Can you work these out from the model? Positions are in its coordinate system, mm. Face numbers are marked on the shaded views. A direction names the side the tool comes from. Coordinates: 2 decimals unless noted, no trailing zeros. Loops run counter-clockwise (first coordinate to the right, second up) from the corner with the lowest first, then second, coordinate; pieces in that order, holes last.
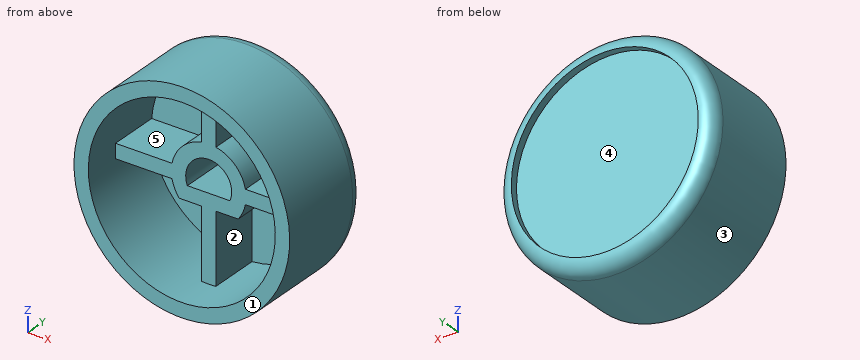
```python
from build123d import *

# Parameters (mm, degrees)
SKETCH1_R           = 15
BOSS_EXTRUDE1_DEPTH = 14.2
SHELL1_T            = -2
EXTRUDE_THIN2_DEPTH = 7
RIB1_REACH          = 25.043
SKETCH3_WALLS_W     = 2
SKETCH3_WALLS_H     = 57.886874488
CIRPATTERN1_COUNT   = 4
FILLET1_R           = 2
SKETCH4_R           = 13
CUT_EXTRUDE1_DEPTH  = 1


with BuildPart() as part:
    # Sketch1 → Boss-Extrude1 (new body)
    with BuildSketch(Plane(origin=(0, 0, 0), x_dir=(1, 0, 0), z_dir=(0, 1, 0))):
        with Locations(Location((0, 0, 0), (0, 0, 270))):
            Circle(SKETCH1_R)
    extrude(amount=-BOSS_EXTRUDE1_DEPTH)

    # Shell1
    shell1_openings = [part.faces().sort_by_distance(p)[0] for p in [
        (0, -14.2, 0),
    ]]
    offset(amount=SHELL1_T, openings=shell1_openings, kind=Kind.INTERSECTION)

    # Sketch2 → Extrude-Thin2 (add)
    with BuildSketch(Plane.XZ.offset(2)):
        with BuildLine():
            Line((-4.098780306, -3.2), (4.098780306, -3.2))
            ThreePointArc((4.098780306, -3.2), (0, 5.2), (-4.098780306, -3.2))
        make_face()
        with BuildLine():
            Line((-2.966479395, -1.2), (2.966479395, -1.2))
            ThreePointArc((2.966479395, -1.2), (0, 3.2), (-2.966479395, -1.2))
        make_face(mode=Mode.SUBTRACT)
    extrude(amount=EXTRUDE_THIN2_DEPTH)

    # Sketch3 walls → Rib1 (add, up to next)
    with BuildSketch(Plane.XZ.offset(9), mode=Mode.PRIVATE) as rib1_sk1:
        with Locations((0, -8.1)):
            Rectangle(SKETCH3_WALLS_W, SKETCH3_WALLS_H)
    rib1_tool1 = extrude(rib1_sk1.sketch, amount=-RIB1_REACH, mode=Mode.PRIVATE) - part.part
    rib1 = rib1_tool1.solids().sort_by_distance((0, -9, -8.1))[0]
    add(rib1)

    # CirPattern1: Rib1 ×4 about axis
    cirpattern1_axis = Axis((0, 0, 0), (0, 1, 0))
    for i in range(1, CIRPATTERN1_COUNT):
        add(rib1.rotate(cirpattern1_axis, i * 360 / CIRPATTERN1_COUNT))

    # Fillet1
    fillet1_edges = [part.edges().sort_by_distance(p)[0] for p in [
        (0, 0, -15),
    ]]
    fillet(fillet1_edges, radius=FILLET1_R)

    # Sketch4 → Cut-Extrude1 (cut)
    with BuildSketch(Plane(origin=(0, 0, 0), x_dir=(1, 0, 0), z_dir=(0, 1, 0))):
        with Locations(Location((0, 0, 0), (0, 0, 270))):
            Circle(SKETCH4_R)
    extrude(amount=-CUT_EXTRUDE1_DEPTH, mode=Mode.SUBTRACT)


solid = part.part
```
(1) I want a section at B-B on z = 0. Write out the boundary of the cut face in (x, y).
Check values:
outline: (-15, -14.2) - (-13, -14.2) - (-13, -9) - (-3.2, -9) - (-3.2, -2) - (3.2, -2) - (3.2, -9) - (13, -9) - (13, -14.2) - (15, -14.2) - (15, -2) arc R2 ccw to (13, 0) - (13, -1) - (-13, -1) - (-13, 0) arc R2 ccw to (-15, -2) - close
(2) I'm going to push flat-ended pins straight in: pin 1 (1.5 mm diameter, centred on x = 7.5, y = -12, fed in from +Z); pin 2 (13 mm diameter, centred on x = 6, z = -4.5, fed in from -Y); pin 3 (2 mm diameter, centred on x = -8.5, y = -4.5, fed in from -Z); pin 4 (8 mm diameter, centred on y = -2.5, z = 11.5, fed in from +X). Where does each tip first touch, or does it pass through?
Check values:
pin 1: stops at z = 13.4
pin 2: stops at y = -14.2
pin 3: stops at z = -12.99
pin 4: stops at x = 12.99
(3) Which directions (+Z, -Z, +X, -X, +Y, -Y) give clear straight access to the entire face, cutting with the end or side of a thin tool? Please do the marked faces 4 and 5.
Check values:
face 4: +Y
face 5: -Y
(4) I want a section at C-C on x = 0. Write out the boundary of the cut face in (y, z), then the cut area to 3 significant figures.
Check values:
outline: (-14.2, -15) - (-2, -15) arc R2 ccw to (0, -13) - (-1, -13) - (-1, 13) - (0, 13) arc R2 ccw to (-2, 15) - (-14.2, 15) - (-14.2, 13) - (-9, 13) - (-9, 3.2) - (-2, 3.2) - (-2, -1.2) - (-9, -1.2) - (-9, -13) - (-14.2, -13) - close
area: 232 mm2
(5) If we mould it in two halves opening along X, with no side actions, what happens to the marked faces 1, 2 and 3? For each: released by +X, released by -X, zero draft, split by the parting line, or undercut.
Check values:
face 1: zero draft
face 2: undercut
face 3: split by the parting line
(6) I want a section at A-A on y = -5. Write out the boundary of the cut face in (x, z), then the cut area to 3 significant figures.
Check values:
outline: circle Ø30 at (0, 0); hole (-12.96, -1) arc R13 ccw to (-1, -12.96) - (-1, -3.2) - (-4.1, -3.2) arc R5.2 cw to (-5.1, -1) - close; hole (-12.96, 1) - (-5.1, 1) arc R5.2 cw to (-1, 5.1) - (-1, 12.96) arc R13 ccw to start; hole (-2.97, -1.2) - (2.97, -1.2) arc R3.2 ccw (long way) to start; hole (1, -12.96) arc R13 ccw to (12.96, -1) - (5.1, -1) arc R5.2 cw to (4.1, -3.2) - (1, -3.2) - close; hole (1, 5.1) arc R5.2 cw to (5.1, 1) - (12.96, 1) arc R13 ccw to (1, 12.96) - close
area: 292 mm2
(7) I want a section at D-D on y = -11.5. Write out the boundary of the cut face in (x, z), then the cut area to 3 significant figures.
Check values:
outline: circle Ø30 at (0, 0); hole circle Ø26 at (0, 0)
area: 176 mm2
(8) If I drill on probe 1 along X at (y, z) = (-4.75, 0); probe 2 along X at (y, z) = (-8, 3.25); probe 3 along Z at (x, y) = (0.25, -7.75), over which ranges is the centre line in solid material (lowest first)?
Check values:
probe 1: x = -15 to -3.2, 3.2 to 15
probe 2: x = -14.64 to -12.59, -4.06 to 4.06, 12.59 to 14.64
probe 3: z = -15 to -1.2, 3.19 to 15
